For this review, take the finished solid that the model builds, in its own axes (mm). Face numbers are marked on the shaded views. A direction names the side the tool comes from. Give positions to 0.01 mm unless a question says otherwise; leave off trailing zeros. Order: outer loops, then holes, each group sorted by start corner. A loop starts at its lowest first (then second) coordinate and runs counter-clockwise, first axis right, second up. Notation, with made-up numbers: M 32.25,4 L 66.25,4 A21 ccw 66.25,41 Z; hole C 50.5,32.5 d3. An arc over 180 degrees is marked long. Answer as CSV lines item,"result". Start each with the question number.
1. Mouldability with a two-part tool opening along Y and no side actions: class the marked faces 1, 2 and 3 as pulls with the +Y half, pulls with the -Y half, needs draft (parallel to the pull), parting line crosses it, or undercut.
2. Clearance check with flat-ended pins moving along their axes: P1, Ø4, axis at x = -8.5, y = -8, coming from the -Z side; P2, Ø3, axis at x = 7, z = 7, coming from the +Y side; P3, Ø5, axis at x = -5, z = 2.5, coming from the +Y side; P4, Ø2, axis at x = 1.5, z = 9, coming from the -Y side. State where each tip first meets the part, or that it passes through.
3. We need section A-A, the plane x = 0. Give the boundary of the cut face in (y, z).
4. We need section D-D, the plane z = 11.25. Give the boundary of the cut face in (x, y), and give its area (3 significant figures).
5. For line 1 along Y through (x, z) = (0, 4); line 2 along Z through (x, y) = (-8, 9.5); line 3 along X through (y, z) = (-0.25, 1.5), list the stretches that pass through material, from the lowest coordinate up.
6. Machinability: for the marked faces 4 and 5, which of the approach directions +Z, -Z, +X, -X, +Y, -Y give a long, thin tool a straight path to every point of the face, cutting with its end or side? Answer none if there is none.
7. We need section C-C, the plane z = 1. Give the boundary of the cut face in (x, y), and give its area (3 significant figures).
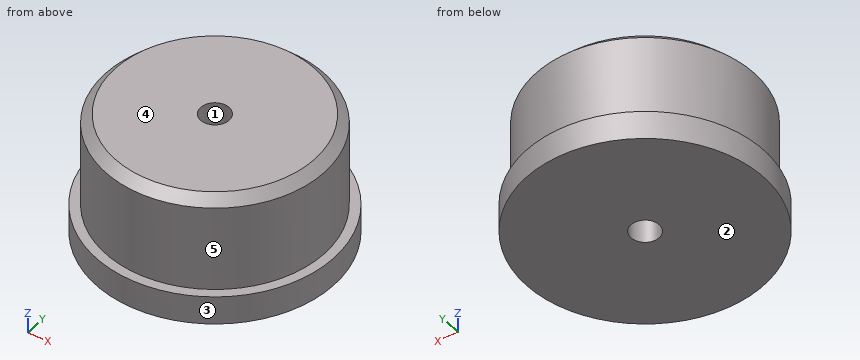
from build123d import *

# Parameters (mm, degrees)
ESQUISSE1_R       = 12.5
EXTRUSION1_DEPTH  = 3
ESQUISSE2_R       = 11.5
EXTRUSION2_DEPTH  = 10
CHANFREIN1_SIZE   = 1
TROU_TARAUD_M41_D = 3


with BuildPart() as part:
    # Esquisse1 → Extrusion1 (new body)
    with BuildSketch(Plane.XY):
        Circle(ESQUISSE1_R)
    extrude(amount=EXTRUSION1_DEPTH)

    # Esquisse2 → Extrusion2 (add)
    with BuildSketch(Plane.XY.offset(3)):
        Circle(ESQUISSE2_R)
    extrude(amount=EXTRUSION2_DEPTH)

    # Chanfrein1
    chanfrein1_edges = [part.edges().sort_by_distance(p)[0] for p in [
        (-11.5, 0, 13),
    ]]
    chamfer(chanfrein1_edges, length=CHANFREIN1_SIZE)

    # Trou taraudé M41 (through all)
    with Locations(Plane(origin=(0, 0, 0), x_dir=(-1, 0, 0), z_dir=(0, 0, -1))):
        with Locations((0, 0)):
            Hole(TROU_TARAUD_M41_D / 2)


solid = part.part
Result set:
1,face 1,"undercut"
1,face 2,"needs draft"
1,face 3,"parting line crosses it"
2,P1,"z = 0"
2,P2,"y = 10.1"
2,P3,"y = 12.25"
2,P4,"y = -11.49"
3,outline,"M -12.5,0 L -1.5,0 L -1.5,13 L -10.5,13 L -11.5,12 L -11.5,3 L -12.5,3 Z; M 1.5,0 L 12.5,0 L 12.5,3 L 11.5,3 L 11.5,12 L 10.5,13 L 1.5,13 Z"
4,outline,"C 0,0 d23; hole C 0,0 d3"
4,area,"408 mm2"
5,line 1,"-11.5 to -1.5, 1.5 to 11.5"
5,line 2,"0 to 3"
5,line 3,"-12.5 to -1.48, 1.48 to 12.5"
6,face 4,"+Z, +X, -X, +Y, -Y"
6,face 5,"+Z"
7,outline,"C 0,0 d25; hole C 0,0 d3"
7,area,"484 mm2"
